Check sheet for the modelled part. Datum: model origin and axes. Units: mm. Face numbers are marked on the shaded views. A direction names the side the tool comes from. Coordinates: 2 decimals unless noted, no trailing zeros. Loops run counter-clockwise (first coordinate to the right, second up) from the corner with the lowest first, then second, coordinate; pieces in that order, holes last. Notation, with made-up numbers: M 31.25,88.25 L 88.25,88.25 A22 cw 88.25,95.25 Z; hole C -34,4 d10. An arc over 180 degrees is marked long. Write each question's results on one line, items separated by ' | '. Start each with the question number.
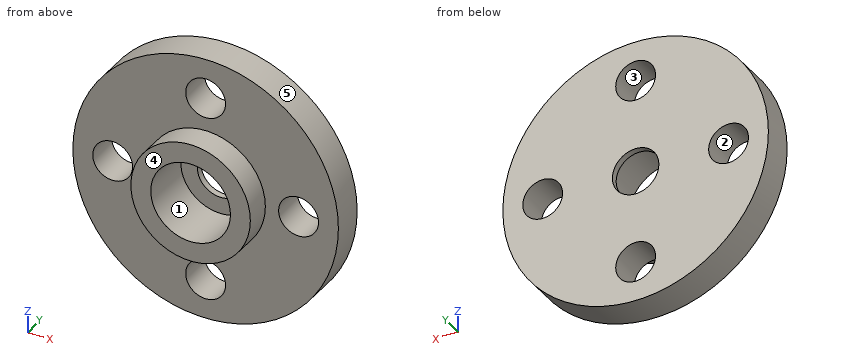
from build123d import *

# Parameters (mm, degrees)
SKETCH1_R           = 10
BOSS_EXTRUDE1_DEPTH = 2.5
SKETCH2_R           = 4.5
SKETCH2_R_2         = 3
BOSS_EXTRUDE2_DEPTH = 2
SKETCH3_R           = 1.5
SKETCH3_R_2         = 1.75
CUT_EXTRUDE1_DEPTH  = 5.5
SKETCH2_2_R         = 3
CUT_EXTRUDE2_DEPTH  = 2


with BuildPart() as part:
    # Sketch1 → Boss-Extrude1 (new body)
    with BuildSketch(Plane(origin=(0, 0, 0), x_dir=(1, 0, 0), z_dir=(0, 1, 0))):
        Circle(SKETCH1_R)
    extrude(amount=BOSS_EXTRUDE1_DEPTH)

    # Sketch2 → Boss-Extrude2 (add)
    with BuildSketch(Plane.XZ):
        Circle(SKETCH2_R)
        Circle(SKETCH2_R_2, mode=Mode.SUBTRACT)
    extrude(amount=BOSS_EXTRUDE2_DEPTH)

    # Sketch3 → Cut-Extrude1 (cut, through all)
    with BuildSketch(Plane(origin=(0, 2.5, 0), x_dir=(1, 0, 0), z_dir=(0, 1, 0))):
        with Locations((0, 7)):
            Circle(SKETCH3_R)
        with Locations((7, 0)):
            Circle(SKETCH3_R)
        with Locations((0, -7)):
            Circle(SKETCH3_R)
        with Locations((-7, 0)):
            Circle(SKETCH3_R)
        Circle(SKETCH3_R_2)
    extrude(amount=-CUT_EXTRUDE1_DEPTH, mode=Mode.SUBTRACT)

    # Sketch2_2 → Cut-Extrude2 (cut)
    with BuildSketch(Plane.XZ):
        Circle(SKETCH2_2_R)
    extrude(amount=-CUT_EXTRUDE2_DEPTH, mode=Mode.SUBTRACT)


solid = part.part
1) Section check A-A (x = 0). Enter the section's corners in (y, z).
2) Section check C-C (z = 7). Enter the section's corners in (x, y).
3) Thickness scan on probe 1 along Z at (x, y) = (0, 0.6); probe 2 along Y at (x, z) = (8.25, 5); probe 3 along X at (y, z) = (1.5, -7). Record the ranges inside material, lowest first.
4) Section check D-D (y = 0.55). Enter the section's corners in (x, z).
5) Release check for a two-part mould opening along Z. For the marked faces 3, 4 and 5 record: +Z half, -Z half, draft (parallel to the pull), parting line (faces both ways), or undercut.
6) Section check B-B (z = 0). Enter the section's corners in (x, y), then the cut area to 4 significant figures.
7) Set-up check for the marked faces 1 and 2: record each of +Z, -Z, +X, -X, +Y, -Y from which the full face is reachable in a straight line by a thin tool's end or side.
8) Gauge pin test, flat ends, axial feed: P1, Ø1.5, axis at y = 0, z = -7.5, coming from the +X side; P2, Ø2, axis at x = -3, y = 0.5, coming from the -Z side; P3, Ø3.5, axis at x = -7, z = 0, coming from the -Y side. Record the tip position at first contact, or that the pin passes through.
Return value:
1) outline: M -2,-4.5 L 0,-4.5 L 0,-5.5 L 2.5,-5.5 L 2.5,-1.75 L 2,-1.75 L 2,-3 L -2,-3 Z; M -2,3 L 2,3 L 2,1.75 L 2.5,1.75 L 2.5,5.5 L 0,5.5 L 0,4.5 L -2,4.5 Z; M 0,-10 L 2.5,-10 L 2.5,-8.5 L 0,-8.5 Z; M 0,8.5 L 2.5,8.5 L 2.5,10 L 0,10 Z
2) outline: M -7.14,0 L -1.5,0 L -1.5,2.5 L -7.14,2.5 Z; M 1.5,0 L 7.14,0 L 7.14,2.5 L 1.5,2.5 Z
3) probe 1: z = -10 to -8.5, -5.5 to -3, 3 to 5.5, 8.5 to 10 | probe 2: y = 0 to 2.5 | probe 3: x = -7.14 to -1.5, 1.5 to 7.14
4) outline: C 0,0 d20; hole C -7,0 d3; hole C 0,0 d6; hole C 0,-7 d3; hole C 0,7 d3; hole C 7,0 d3
5) face 3: undercut | face 4: draft | face 5: parting line
6) outline: M -10,0 L -8.5,0 L -8.5,2.5 L -10,2.5 Z; M -5.5,0 L -4.5,0 L -4.5,-2 L -3,-2 L -3,2 L -1.75,2 L -1.75,2.5 L -5.5,2.5 Z; M 1.75,2 L 3,2 L 3,-2 L 4.5,-2 L 4.5,0 L 5.5,0 L 5.5,2.5 L 1.75,2.5 Z; M 8.5,0 L 10,0 L 10,2.5 L 8.5,2.5 Z | area: 27.25 mm2
7) face 1: -Y | face 2: +Y, -Y
8) P1: stops at x = 7.38 | P2: stops at z = -9.8 | P3: stops at y = 0
